Verification items for the finished model (mm, model axes). Face numbers are marked on the shaded views. A direction names the side the tool comes from. Coordinates: 2 decimals unless noted, no trailing zeros. Loops run counter-clockwise (first coordinate to the right, second up) from the corner with the lowest first, then second, coordinate; pieces in that order, holes last.
Q1. Sectioned sample at C-C (x = 2). Enter the section's corners in (y, z).
Q2. Go/stop test with flat-tipped pins: P1, Ø1.5, axis at y = 2, z = 5.5, coming from the -X side; P2, Ø1, axis at y = 1, z = 2, coming from the -X side; P3, Ø1.5, axis at y = 1.5, z = 2, coming from the +X side; P4, Ø1, axis at x = 1, z = 4, coming from the -Y side. Record where each tip stops, or that it passes through.
Q3. Material ranges on probe 1 along X at (y, z) = (1.7, 2.25); probe 2 along X at (y, z) = (2.4, 0.5); probe 3 along Y at (x, z) = (0.25, 5.5), recorded low to high.
Q4. Mould release check, pull along X, two halves, no side actions. Record for the marked faces 3, 4, 5 and 6: +X half, -X half, draft (parallel to the pull), parting line (faces both ways), or undercut.
Q5. Sectioned sample at B-B (y = 2.1). Enter the section's corners in (x, z), then the cut area to 3 significant figures.
Q6. Sectioned sample at D-D (x = -0.75). Enter the section's corners in (y, z), then the cut area to 3 significant figures.
Q7. Sectioned sample at A-A (z = 1). Enter the section's corners in (x, y).
Q8. Access from +Z, -Z, +X, -X, +Y, -Y to the whole of each face (thin tool, end or side, straight path). Record for the marked faces 1 and 2.
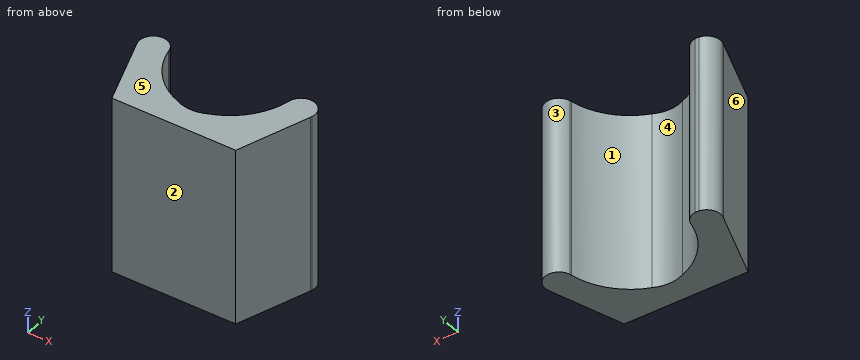
```python
from build123d import *

# Parameters (mm, degrees)
F1_DEPTH = 6.53


with BuildPart() as f1:
    # F0 (on Top) → F1 (new body)
    with BuildSketch(Plane.XY):
        with BuildLine():
            Line((-2.25, 0), (0, 0))
            Line((0, 0), (2.25, 0))
            Line((2.25, 0), (3.156994, 2.602679))
            Line((3.156994, 2.602679), (3.173864, 2.651089))
            ThreePointArc((3.173864, 2.651089), (2.825283, 3.284668), (2.193543, 2.932764))
            ThreePointArc((2.193543, 2.932764), (2.186252, 2.895291), (2.178403, 2.85793))
            ThreePointArc((2.178403, 2.85793), (1.604596, 1.718806), (0.551908, 0.998591))
            ThreePointArc((0.551908, 0.998591), (0, 0.87272), (-0.551908, 0.998591))
            ThreePointArc((-0.551908, 0.998591), (-1.604596, 1.718806), (-2.178403, 2.85793))
            ThreePointArc((-2.178403, 2.85793), (-2.186252, 2.895291), (-2.193543, 2.932764))
            ThreePointArc((-2.193543, 2.932764), (-2.350233, 3.179732), (-2.616842, 3.3))
            Line((-2.616842, 3.3), (-2.752045, 3.3))
            ThreePointArc((-2.752045, 3.3), (-3.112041, 3.072457), (-3.173864, 2.651089))
            Line((-3.173864, 2.651089), (-3.156994, 2.602679))
            Line((-3.156994, 2.602679), (-2.25, 0))
        make_face()
        with BuildLine():
            ThreePointArc((-3.173864, 2.651089), (-3.166038, 2.626672), (-3.156994, 2.602679))
            Line((-3.156994, 2.602679), (-3.173864, 2.651089))
        make_face()
        with BuildLine():
            Line((3.173864, 2.651089), (3.156994, 2.602679))
            ThreePointArc((3.156994, 2.602679), (3.166038, 2.626672), (3.173864, 2.651089))
        make_face()
        with BuildLine():
            ThreePointArc((-2.616842, 3.3), (-2.684443, 3.3045), (-2.752045, 3.3))
            Line((-2.752045, 3.3), (-2.616842, 3.3))
        make_face()
        with BuildLine():
            ThreePointArc((2.178403, 2.85793), (2.186252, 2.895291), (2.193543, 2.932764))
            ThreePointArc((2.193543, 2.932764), (2.18457, 2.895631), (2.178403, 2.85793))
        make_face()
        with BuildLine():
            ThreePointArc((-2.178403, 2.85793), (-2.18457, 2.895631), (-2.193543, 2.932764))
            ThreePointArc((-2.193543, 2.932764), (-2.186252, 2.895291), (-2.178403, 2.85793))
        make_face()
    extrude(amount=F1_DEPTH)


solid = f1.part
```
Geometry check:
1. outline: (0, 0) - (2.33, 0) - (2.33, 6.53) - (0, 6.53) - close
2. P1: stops at x = -3.19
2. P2: stops at x = -2.77
2. P3: stops at x = 3.03
2. P4: stops at y = 0
3. probe 1: x = -2.84 to -1.59, 1.59 to 2.84
3. probe 2: x = -3.09 to -2.03, 2.03 to 3.09
3. probe 3: y = 0 to 0.9
4. face 3: undercut
4. face 4: undercut
4. face 5: draft
4. face 6: -X half
5. outline: (-2.98, 0) - (-1.88, 0) - (-1.88, 6.53) - (-2.98, 6.53) - close; (1.88, 0) - (2.98, 0) - (2.98, 6.53) - (1.88, 6.53) - close
5. area: 14.4 mm2
6. outline: (0, 0) - (1.08, 0) - (1.08, 6.53) - (0, 6.53) - close
6. area: 7.05 mm2
7. outline: (-3.17, 2.65) arc R0.51 ccw to (-3.16, 2.6) - (-2.25, 0) - (2.25, 0) - (3.16, 2.6) arc R0.51 ccw to (3.17, 2.65) arc R0.51 ccw (long way) to (2.19, 2.93) arc R0.51 ccw to (2.18, 2.86) arc R2.56 cw to (0.55, 1) arc R1.27 cw to (-0.55, 1) arc R2.56 cw to (-2.18, 2.86) arc R0.51 ccw to (-2.19, 2.93) arc R0.51 ccw to (-2.62, 3.3) arc R0.51 ccw to (-2.75, 3.3) arc R0.51 ccw to start
8. face 1: +Z, -Z, +Y
8. face 2: +Z, -Z, +X, -X, -Y
